Here's how the part is built. I have some questions about the finished solid (model axes, mm). Face numbers are marked on the shaded views. A direction names the side the tool comes from. Give positions to 0.01 mm unless a question says otherwise; leave off trailing zeros. Order: outer loops, then holes, each group sorted by start corner. A loop starts at its lowest first (then second) coordinate and runs counter-clockwise, first axis right, second up. Notation, with made-up numbers: M 81.5,-27 L 121.5,-27 A17 cw 121.5,-14 Z; hole C -37.75,-1 d3. An arc over 180 degrees is marked long. One line per item, written item: value. Start each with the question number.
from build123d import *

# Parameters (mm, degrees)
BOSS_EXTRUDE1_DEPTH = 6.35
SKETCH2_R           = 1.35
SKETCH2_R_2         = 1.385
CUT_EXTRUDE1_DEPTH  = 38.116505762
SKETCH3_W           = 63.5
SKETCH3_H           = 88.9
SKETCH3_W_2         = 38.321076004
SKETCH3_H_2         = 47.237540142
BOSS_EXTRUDE2_DEPTH = 6.35
SKETCH5_W           = 27.94
SKETCH5_H           = 55.88
CUT_EXTRUDE3_DEPTH  = 61.153053743
SKETCH6_R           = 3.175
CUT_EXTRUDE4_DEPTH  = 61.153053743
FILLET2_R           = 7.62


with BuildPart() as part:
    # Sketch1 → Boss-Extrude1 (new body)
    with BuildSketch(Plane.XY):
        with BuildLine():
            Line((-19.69889026, 23.2987845), (-14.850045261, 29.75147823))
            ThreePointArc((-14.850045261, 29.75147823), (-14.144755454, 30.339267512), (-13.251155001, 30.55))
            Line((-13.251155001, 30.55), (13.251155001, 30.55))
            ThreePointArc((13.251155001, 30.55), (14.144755454, 30.339267512), (14.850045261, 29.75147823))
            Line((14.850045261, 29.75147823), (19.69889026, 23.2987845))
            ThreePointArc((19.69889026, 23.2987845), (19.997074131, 22.730638521), (20.1, 22.09730627))
            Line((20.1, 22.09730627), (20.1, -22.09730627))
            ThreePointArc((20.1, -22.09730627), (19.997074131, -22.730638521), (19.69889026, -23.2987845))
            Line((19.69889026, -23.2987845), (14.850045261, -29.75147823))
            ThreePointArc((14.850045261, -29.75147823), (14.144755454, -30.339267512), (13.251155001, -30.55))
            Line((13.251155001, -30.55), (-13.251155001, -30.55))
            ThreePointArc((-13.251155001, -30.55), (-14.144755454, -30.339267512), (-14.850045261, -29.75147823))
            Line((-14.850045261, -29.75147823), (-19.69889026, -23.2987845))
            ThreePointArc((-19.69889026, -23.2987845), (-19.997074131, -22.730638521), (-20.1, -22.09730627))
            Line((-20.1, -22.09730627), (-20.1, 22.09730627))
            ThreePointArc((-20.1, 22.09730627), (-19.997074131, 22.730638521), (-19.69889026, 23.2987845))
        make_face()
    extrude(amount=-BOSS_EXTRUDE1_DEPTH)

    # Sketch2 → Cut-Extrude1 (cut, through all)
    with BuildSketch(Plane(origin=(0, 0, -6.35), x_dir=(-1, 0, 0), z_dir=(0, 0, -1))):
        with Locations((17.3, 21.9487845)):
            Circle(SKETCH2_R)
        with Locations((17.3, -0.0512155)):
            Circle(SKETCH2_R)
        with Locations((17.3, -22.0512155)):
            Circle(SKETCH2_R)
        with Locations((11, -27.75)):
            Circle(SKETCH2_R_2)
        with Locations(Location((-11, -27.75, 0), (0, 0, 180))):
            Circle(SKETCH2_R_2)
        with Locations(Location((-17.3, -22.0512155, 0), (0, 0, 180))):
            Circle(SKETCH2_R)
        with Locations(Location((-17.3, -0.0512155, 0), (0, 0, 180))):
            Circle(SKETCH2_R)
        with Locations(Location((-17.3, 21.9487845, 0), (0, 0, 180))):
            Circle(SKETCH2_R)
    extrude(amount=-CUT_EXTRUDE1_DEPTH, mode=Mode.SUBTRACT)

    # Sketch3 → Boss-Extrude2 (add)
    with BuildSketch(Plane(origin=(0, 0, -6.35), x_dir=(-1, 0, 0), z_dir=(0, 0, -1))):
        with Locations((0, -6.2452155)):
            Rectangle(SKETCH3_W, SKETCH3_H)
        Rectangle(SKETCH3_W_2, SKETCH3_H_2, mode=Mode.SUBTRACT)
    extrude(amount=-BOSS_EXTRUDE2_DEPTH)

    # Sketch5 → Cut-Extrude3 (cut, through all)
    with BuildSketch(Plane.XY):
        with Locations((0, 3.0087845)):
            Rectangle(SKETCH5_W, SKETCH5_H)
    extrude(amount=-CUT_EXTRUDE3_DEPTH, mode=Mode.SUBTRACT)

    # Sketch6 → Cut-Extrude4 (cut, through all)
    with BuildSketch(Plane(origin=(0, 0, -6.35), x_dir=(-1, 0, 0), z_dir=(0, 0, -1))):
        with Locations((25.4, 31.8547845)):
            Circle(SKETCH6_R)
        with Locations((-25.4, 31.8547845)):
            Circle(SKETCH6_R)
        with Locations((-25.4, -36.7252155)):
            Circle(SKETCH6_R)
        with Locations((25.4, -36.7252155)):
            Circle(SKETCH6_R)
    extrude(amount=-CUT_EXTRUDE4_DEPTH, mode=Mode.SUBTRACT)

    # Fillet2
    fillet2_edges = [part.edges().sort_by_distance(p)[0] for p in [
        (-31.75, 38.2047845, -3.175),
        (-31.75, -50.6952155, -3.175),
        (31.75, -50.6952155, -3.175),
        (31.75, 38.2047845, -3.175),
    ]]
    fillet(fillet2_edges, radius=FILLET2_R)


solid = part.part
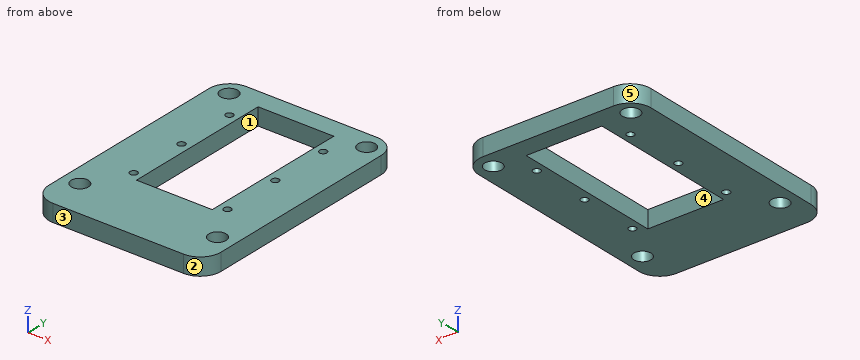
Item 1: For the marked faces 1 and 2, which set-ups out of +Z, -Z, +X, -X, +Y, -Y let a thin tool reach every point of the face, with its end or its side?
Item 2: Please list where these lines run through material, in increasing order: probe 1 along Y at (x, z) = (17.3, -1.5); probe 2 along X at (y, z) = (-8, -4.5); probe 3 along X at (y, z) = (-34, -5.75). Write a range as [from, to].
Item 3: I want a section at C-C on x = -17.3. Write out the boundary of the cut face in (y, z), plus the area to 3 significant figures.
Item 4: Will this pin go through, and if not, where does the flat tip stop? P1, Ø2, axis at x = -17.3, y = -0.05, coming from the +Z side.
Item 5: I want a section at D-D on z = -4. Count the separate pieces of the cut face and the enclosed holes in it, plus the area to 3 significant figures.
Item 6: We'd pull the mould along X, two halves only. Please class the marked faces 3, 4 and 5: +X half, -X half, draft (parallel to the pull), parting line (faces both ways), or undercut.
Item 7: I want a section at A-A on x = -3. Write out the boundary of the cut face in (y, z).
Item 8: I want a section at B-B on y = -14. Write out the boundary of the cut face in (x, z).
Answer below:
1. face 1: +Z, -Z
1. face 2: +Z, -Z, +X, -Y
2. probe 1: y = [-50.7, -23.4], [-20.7, -1.4], [1.3, 20.6], [23.3, 38.2]
2. probe 2: x = [-31.75, -13.97], [13.97, 31.75]
2. probe 3: x = [-31.75, -27.03], [-23.77, 23.77], [27.03, 31.75]
3. outline: M -50.7,-6.35 L -23.4,-6.35 L -23.4,0 L -50.7,0 Z; M -20.7,-6.35 L -1.4,-6.35 L -1.4,0 L -20.7,0 Z; M 1.3,-6.35 L 20.6,-6.35 L 20.6,0 L 1.3,0 Z; M 23.3,-6.35 L 38.2,-6.35 L 38.2,0 L 23.3,0 Z
3. area: 513 mm²
4. P1: passes through
5. separate pieces: 1
5. enclosed holes: 11
5. area: 3,870 mm²
6. face 3: draft
6. face 4: undercut
6. face 5: -X half
7. outline: M -50.7,-6.35 L -24.93,-6.35 L -24.93,0 L -50.7,0 Z; M 30.95,-6.35 L 38.2,-6.35 L 38.2,0 L 30.95,0 Z
8. outline: M -31.75,-6.35 L -13.97,-6.35 L -13.97,0 L -31.75,0 Z; M 13.97,-6.35 L 31.75,-6.35 L 31.75,0 L 13.97,0 Z
